from build123d import *

# Parameters (mm, degrees)
SKETCH1_W           = 184.15
SKETCH1_H           = 309.88
BOSS_EXTRUDE1_DEPTH = 1.5875
SKETCH2_R           = 3.175
CUT_EXTRUDE1_DEPTH  = 181.240753941


with BuildPart() as part:
    # Sketch1 → Boss-Extrude1 (new body)
    with BuildSketch(Plane(origin=(0, 0, 0), x_dir=(1, 0, 0), z_dir=(0, 1, 0))):
        Rectangle(SKETCH1_W, SKETCH1_H)
    extrude(amount=BOSS_EXTRUDE1_DEPTH)

    # Sketch2 → Cut-Extrude1 (cut, through all)
    with BuildSketch(Plane(origin=(0, 1.5875, 0), x_dir=(1, 0, 0), z_dir=(0, 1, 0))):
        with Locations(Location((-73.025, 9.525, 0), (0, 0, 270))):
            Circle(SKETCH2_R)
        with Locations(Location((-73.025, -9.525, 0), (0, 0, 270))):
            Circle(SKETCH2_R)
        with Locations(Location((-73.025, 116.84, 0), (0, 0, 270))):
            Circle(SKETCH2_R)
        with Locations(Location((-73.025, 97.79, 0), (0, 0, 270))):
            Circle(SKETCH2_R)
        with Locations(Location((-73.025, -116.84, 0), (0, 0, 270))):
            Circle(SKETCH2_R)
        with Locations(Location((-73.025, -97.79, 0), (0, 0, 270))):
            Circle(SKETCH2_R)
    cut_extrude1 = extrude(amount=-CUT_EXTRUDE1_DEPTH, mode=Mode.SUBTRACT)

    # Mirror1: Cut-Extrude1 across plane
    add(cut_extrude1.mirror(Plane(origin=(0, 0, 0), x_dir=(0, 0, 1), z_dir=(1, 0, 0))), mode=Mode.SUBTRACT)


solid = part.part
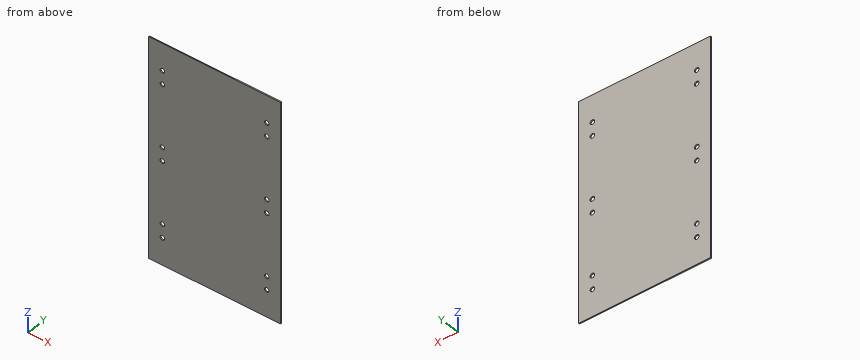
Source: CAD feature listing. Evaluate the final solid. Frame: model axes, mm. Coordinates: 2 decimals unless noted, no trailing zeros. Loops run counter-clockwise (first coordinate to the right, second up) from the corner with the lowest first, then second, coordinate; pieces in that order, holes last. Notation, with made-up numbers: (-7, -40) - (11, -40) arc R23 ccw to (11, -17) - close; hole circle Ø2 at (37, 15.25). An arc over 180 degrees is marked (long way). One line per item, written item: value. Start each with the question number.
1. Ray query, L1, parallel to X at y = 0.6, z = 97.79 (3 decimals). Return the intervals inside material, ascending.
2. Section A-A (z = -116.84). State how many separate pieces and enclosed holes the cut face has, and give its area (3 significant figures).
3. Section B-B (z = 98). Return the cut outline in (x, y) (1 decimal).
Verdict:
1. L1: x = -92.075 to -76.2, -69.85 to 69.85, 76.2 to 92.075
2. separate pieces: 3
2. enclosed holes: 0
2. area: 272 mm2
3. outline: (-92.1, 0) - (-76.2, 0) - (-76.2, 1.6) - (-92.1, 1.6) - close; (-69.9, 0) - (69.9, 0) - (69.9, 1.6) - (-69.9, 1.6) - close; (76.2, 0) - (92.1, 0) - (92.1, 1.6) - (76.2, 1.6) - close
